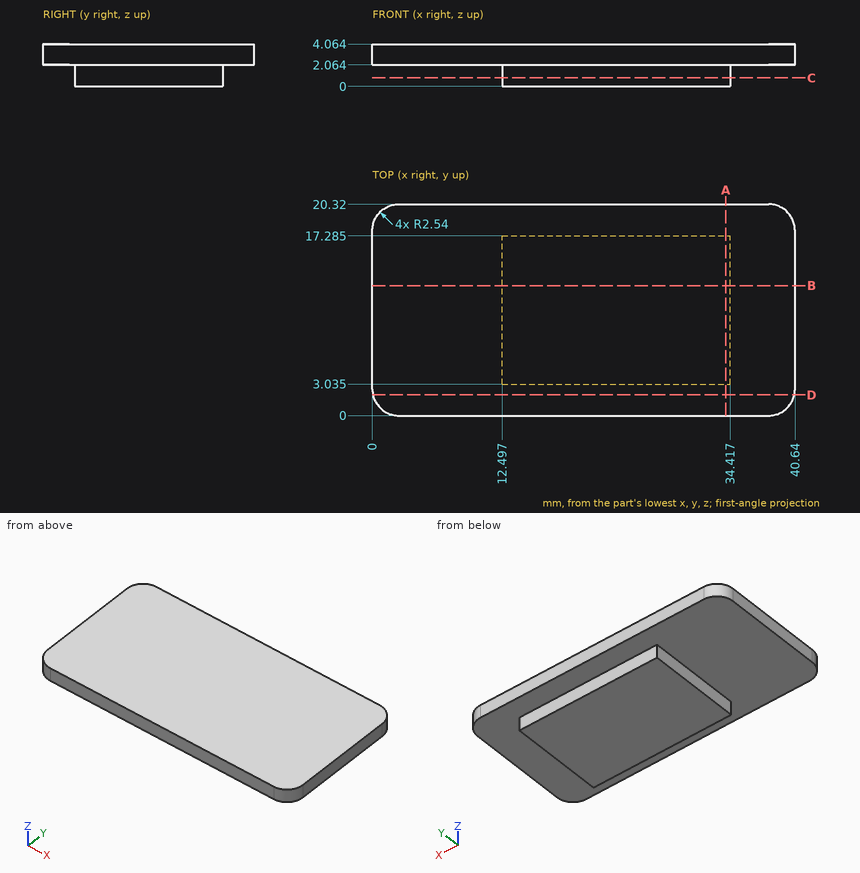
Geometry check sheet. Reference: drawing and pictorial views, mm from the part's lowest x, y, z. Give positions to 0.01 mm unless a question says otherwise; leave off trailing zeros. Loops run counter-clockwise (first coordinate to the right, second up) from the corner with the lowest first, then second, coordinate; pieces in that order, holes last.
1. Section check B-B, the plane y = 12.5. Enter the section's corners in (x, z).
2. Section check D-D, the plane y = 2. Enter the section's corners in (x, z).
3. Go/stop test with flat-tipped pins: pin 1 Ø1 at (x, z) = (28, 1) entering from +Y (1 decimal); pin 2 Ø1 at (x, y) = (11.5, 13) entering from -Z; pin 3 Ø1 at (y, z) = (14.5, 0.5) entering from +X. Record where each tip stops, or that it passes through.
4. Section check A-A, the plane x = 34. Enter the section's corners in (y, z) (1 decimal).
5. Section check C-C, the plane z = 0.8. Enter the section's corners in (x, y) (1 decimal), then the cut area to 3 significant figures.
6. Thickness scan on line 1 (Y direction, x = 19, z = 1.85) (1 decimal); line 2 (Z direction, x = 28, y = 18.5); line 3 (X direction, y = 9.5, z = 0.95). Record the ranges inside material, lowest first.
Geometry says:
1. outline: (0, 2.06) - (12.5, 2.06) - (12.5, 0) - (34.42, 0) - (34.42, 2.06) - (40.64, 2.06) - (40.64, 4.06) - (0, 4.06) - close
2. outline: (0.06, 2.06) - (40.58, 2.06) - (40.58, 4.06) - (0.06, 4.06) - close
3. pin 1: stops at y = 17.3
3. pin 2: stops at z = 2.06
3. pin 3: stops at x = 34.42
4. outline: (0, 2.1) - (3, 2.1) - (3, 0) - (17.3, 0) - (17.3, 2.1) - (20.3, 2.1) - (20.3, 4.1) - (0, 4.1) - close
5. outline: (12.5, 3) - (34.4, 3) - (34.4, 17.3) - (12.5, 17.3) - close
5. area: 312 mm2
6. line 1: y = 3 to 17.3
6. line 2: z = 2.06 to 4.06
6. line 3: x = 12.5 to 34.42
